The figure shows three views and two pictorial views of one solid part (mm, origin at its lowest corner). Answer the questions. A direction names the side the tool comes from. Coordinates: 2 decimals unless noted, no trailing zeros. Write each loop counter-clockwise with the first axis right and the second up, starting at its lowest first coordinate (ties: lowest second). Pieces come first, ordered by that corner, then holes.
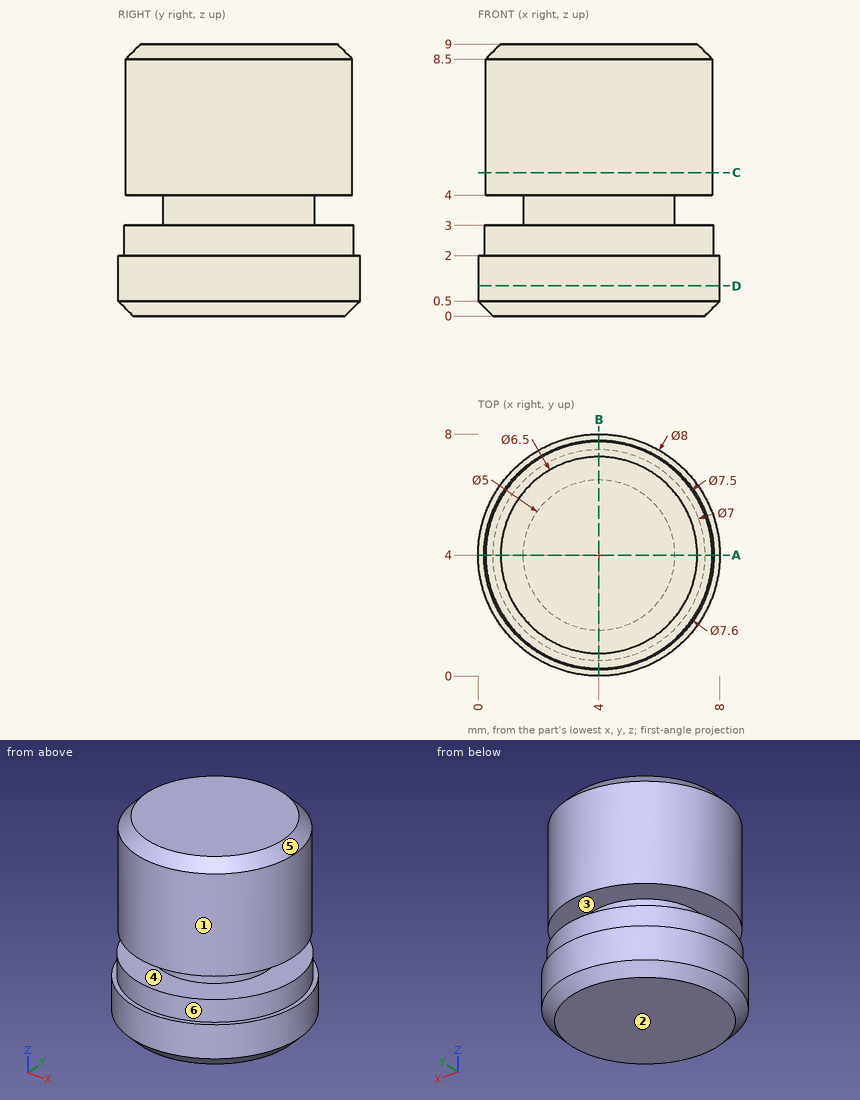
Item 1: The part is cut by section D-D (z = 1). Give the vertices of the cut face in (x, y).
Item 2: The part is cut by section C-C (z = 4.75). Give the vertices of the cut face in (x, y).
Item 3: Determine the mould class of the marked faces 4, 5 and 6 for opening direction Z: +Z half, -Z half, draft (parallel to the pull), parting line (faces both ways), or undercut.
Item 4: For the marked faces 1, 2 and 3, determine the directions among +Z, -Z, +X, -X, +Y, -Y from which every point of the face is accessible in a straight line to the end or side of a thin tool.
Item 5: Given pin 1 (3 mm diameter, centred on x = 5.5, z = 5, fed in from +Y); pin 2 (1.5 mm diameter, centred on y = 2.5, z = 3.5, fed in from +X), each flat-ended and moving along its own axis, determine where each tip first touches the part or whether it passes through.
Item 6: The part is cut by section A-A (y = 4). Give the vertices of the cut face in (x, z), and give its area (3 significant figures).
Item 7: Find the intervals of material crossed by probe 1 along Z at (x, y) = (3, 0.75); probe 2 along Y at (x, z) = (4, 7.5); probe 3 along Y at (x, z) = (6, 4.25), in increasing order.
Answer:
1. outline: circle Ø8 at (4, 4)
2. outline: circle Ø7.5 at (4, 4)
3. face 4: undercut
3. face 5: +Z half
3. face 6: draft
4. face 1: +Z
4. face 2: -Z, +X, -X, +Y, -Y
4. face 3: none
5. pin 1: stops at y = 7.75
5. pin 2: stops at x = 7.68
6. outline: (0, 0.5) - (0.5, 0) - (7.5, 0) - (8, 0.5) - (8, 2) - (7.8, 2) - (7.8, 3) - (6.5, 3) - (6.5, 4) - (7.75, 4) - (7.75, 8.5) - (7.25, 9) - (0.75, 9) - (0.25, 8.5) - (0.25, 4) - (1.5, 4) - (1.5, 3) - (0.2, 3) - (0.2, 2) - (0, 2) - close
6. area: 65.6 mm2
7. probe 1: z = 0 to 3, 4 to 8.85
7. probe 2: y = 0.25 to 7.75
7. probe 3: y = 0.83 to 7.17
